Can you work these out from the model? Positions are in its coordinate system, mm. Give positions to 0.01 mm unless a question says otherwise; leave off trailing zeros. Order: outer loops, then holes, each group sorted by start corner. A loop starts at its lowest first (then second) coordinate and runs counter-clockwise, first axis right, second up. Notation, with made-up numbers: (-37, 64) - (21, 64) arc R29 cw to (21, 91) - close; hole circle Ø7 at (5.5, 22). An arc over 180 degrees is marked (long way). Answer as a JSON object with one key per item and string values.
```python
from build123d import *

# Parameters (mm, degrees)
F0_R     = 2.7
F1_DEPTH = 12.6
F2_R     = 1
F3_R     = 0.25
F4_DEPTH = 12


with BuildPart() as f1:
    # F0 (on Top) → F1 (new body)
    with BuildSketch(Plane.XY):
        Circle(F0_R)
    extrude(amount=F1_DEPTH)

    # F2
    f2_edges = [f1.edges().sort_by_distance(p)[0] for p in [
        (-2.7, 0, 12.6),
    ]]
    fillet(f2_edges, radius=F2_R)

    # F3 (on Top) → F4 (join)
    with BuildSketch(Plane.XY):
        with Locations((-1, 0)):
            Circle(F3_R)
        with Locations((1, 0)):
            Circle(F3_R)
    extrude(amount=-F4_DEPTH)


solid = f1.part
```
Q1. If we section it at A-A, the plane y = 0: Please give me the cut outline in (x, z).
Recorded:
{"outline": "(-2.7, 0) - (-1.25, 0) - (-1.25, -12) - (-0.75, -12) - (-0.75, 0) - (0.75, 0) - (0.75, -12) - (1.25, -12) - (1.25, 0) - (2.7, 0) - (2.7, 11.6) arc R1 ccw to (1.7, 12.6) - (-1.7, 12.6) arc R1 ccw to (-2.7, 11.6) - close"}
Q2. If we section it at B-B, the plane z = -4: Please give me the cut outline in (x, y).
Recorded:
{"outline": "circle Ø0.5 at (-1, 0); circle Ø0.5 at (1, 0)"}
Q3. If we section it at C-C, the plane x = 0: Please give me the cut outline in (y, z).
Recorded:
{"outline": "(-2.7, 0) - (2.7, 0) - (2.7, 11.6) arc R1 ccw to (1.7, 12.6) - (-1.7, 12.6) arc R1 ccw to (-2.7, 11.6) - close"}
Q4. I'm going to push flat-ended pins straight in: pin 1 Ø1 at (y, z) = (1.5, -9.5) entering from -X; pin 2 Ø1.5 at (x, z) = (1.5, 1.5) entering from -Y. Where does each tip first touch, or does it pass through?
Recorded:
{"pin 1": "passes through", "pin 2": "stops at y = -2.59"}
Q5. I need wall thicknesses on L1, parallel to Z at x = -0.15, y = 0.5; L2, parallel to Y at x = 1, z = -4.25; L3, parallel to X at y = -0.1, z = -3.5. Which ranges of each line are inside material? Lowest first, please.
Recorded:
{"L1": "z = 0 to 12.6", "L2": "y = -0.25 to 0.25", "L3": "x = -1.23 to -0.77, 0.77 to 1.23"}
